Build history of the part. All positions in model axes, mm. Round coordinates to 2 decimals unless told otherwise and drop trailing zeros. Write each loop counter-clockwise with the first axis right and the second up, starting at its lowest first coordinate (ties: lowest second). Pieces come first, ordered by that corner, then holes.
Item 1: Band-saw the part on B-B, the plane z = 793. Write the cut outline in (x, y), then the cut area to 3 significant figures.
Item 2: Band-saw the part on A-A, the plane y = 556. Write the cut outline in (x, z).
Item 3: Drop flat-ended pins along their axis: pin 1 Ø1 at (y, z) = (111, 791.5) entering from +X; pin 2 Ø8 at (y, z) = (292.5, 795.5) entering from +X; pin 3 Ø4 at (y, z) = (532, 794) entering from +X. Give the stop position or say it passes through.
Item 4: Band-saw the part on D-D, the plane y = 302.5. Write the cut outline in (x, z), then the cut area to 3 significant figures.
Item 5: Wall check: probe 1 along Y at (x, z) = (30, 790.5); probe 2 along X at (y, z) = (449.5, 786); probe 3 along X at (y, z) = (473, 791.5). Give the ranges that are in metal, low to high.
Item 6: Band-saw the part on C-C, the plane x = -106. Write the cut outline in (y, z).
```python
from build123d import *

# Parameters (mm, degrees)
F2_DEPTH = 20


with BuildPart() as f2:
    # F1 (on offset) → F2 (new body)
    with BuildSketch(Plane.XY.offset(800)):
        Polygon((-200, 346.410162), (0, 0), (200, 346.410162), align=None)
        Polygon((-1000, 346.410162), (-600, 346.410162), (-800, 692.820323), align=None)
        Polygon((200, 346.410162), (0, 0), (400, 0), align=None)
        Polygon((-200, -346.410162), (0, 0), (-400, 0), align=None)
        Polygon((-800, 0), (-600, 346.410162), (-1000, 346.410162), align=None)
        Polygon((1200, 692.820323), (800, 692.820323), (1000, 346.410162), align=None)
        Polygon((-400, 0), (0, 0), (-200, 346.410162), align=None)
        Polygon((-1000, 346.410162), (-800, 692.820323), (-1200, 692.820323), align=None)
        Polygon((400, 692.820323), (200, 346.410162), (600, 346.410162), align=None)
        Polygon((800, 692.820323), (400, 692.820323), (600, 346.410162), align=None)
        Polygon((1000, 346.410162), (600, 346.410162), (800, 0), align=None)
        Polygon((400, 0), (0, 0), (200, -346.410162), align=None)
        Polygon((200, -346.410162), (0, 0), (-200, -346.410162), align=None)
        Polygon((800, 0), (400, 0), (600, -346.410162), align=None)
        Polygon((600, -346.410162), (400, 0), (200, -346.410162), align=None)
        Polygon((-800, 692.820323), (-600, 346.410162), (-400, 692.820323), align=None)
        Polygon((-600, -346.410162), (-200, -346.410162), (-400, 0), align=None)
        Polygon((-600, -346.410162), (-400, 0), (-800, 0), align=None)
        Polygon((-600, 346.410162), (-200, 346.410162), (-400, 692.820323), align=None)
        Polygon((-400, 0), (-200, 346.410162), (-600, 346.410162), align=None)
        Polygon((600, 346.410162), (200, 346.410162), (400, 0), align=None)
        Polygon((800, 692.820323), (600, 346.410162), (1000, 346.410162), align=None)
        Polygon((-800, 0), (-400, 0), (-600, 346.410162), align=None)
        Polygon((600, 346.410162), (400, 0), (800, 0), align=None)
    extrude(amount=-F2_DEPTH)


solid = f2.part
```
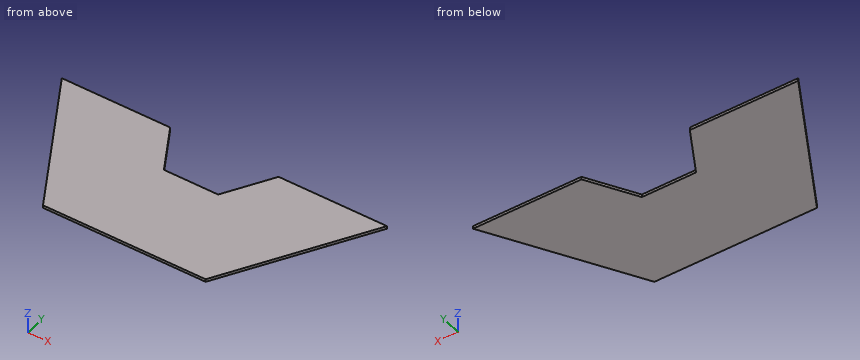
Results:
1. outline: (-1200, 692.82) - (-600, -346.41) - (600, -346.41) - (1200, 692.82) - (400, 692.82) - (200, 346.41) - (-200, 346.41) - (-400, 692.82) - close
1. area: 1,660,000 mm2
2. outline: (-1121.01, 780) - (-321.01, 780) - (-321.01, 800) - (-1121.01, 800) - close; (321.01, 780) - (1121.01, 780) - (1121.01, 800) - (321.01, 800) - close
3. pin 1: stops at x = 864.37
3. pin 2: stops at x = 971.18
3. pin 3: stops at x = 1108.31
4. outline: (-974.65, 780) - (974.65, 780) - (974.65, 800) - (-974.65, 800) - close
4. area: 39,000 mm2
5. probe 1: y = -346.41 to 346.41
5. probe 2: x = -1059.52 to -259.52, 259.52 to 1059.52
5. probe 3: x = -1073.09 to -273.09, 273.09 to 1073.09
6. outline: (-346.41, 780) - (346.41, 780) - (346.41, 800) - (-346.41, 800) - close
